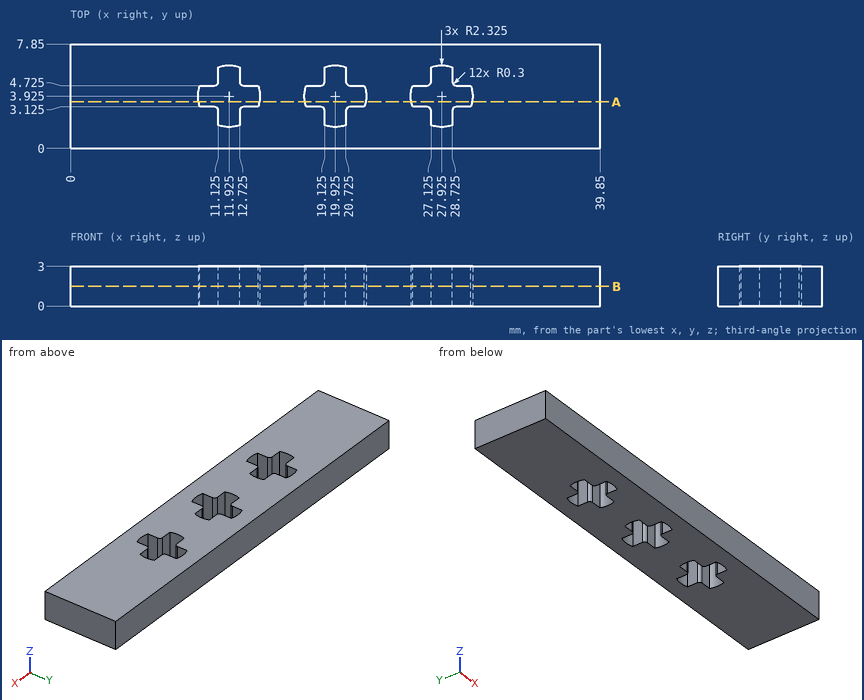
Input: dimensioned drawing with shaded views. Units: mm. Origin: part minimum x, y, z. Give positions to 0.01 mm unless a question says otherwise; leave off trailing zeros. Loops run counter-clockwise (first coordinate to the right, second up) from the corner with the lowest first, then second, coordinate; pieces in that order, holes last. Notation, with made-up numbers: M 87,68 L 138,68 A20 ccw 138,98 Z; hole C 85.25,11.5 d7. An arc over 180 degrees is marked long. Put each result on its own line as item: value.
1) Cut plane A-A, the plane y = 3.5. Return the cut outline in (x, z), plus the area to 3 significant figures.
Computed values:
outline: M 0,0 L 9.64,0 L 9.64,3 L 0,3 Z; M 14.21,0 L 17.64,0 L 17.64,3 L 14.21,3 Z; M 22.21,0 L 25.64,0 L 25.64,3 L 22.21,3 Z; M 30.21,0 L 39.85,0 L 39.85,3 L 30.21,3 Z
area: 78.4 mm^2
2) Material intervals for L1, parallel to X at y = 2.25, z = 1.4 (3 decimals); L2, parallel to X at y = 3.75, z = 0.8; L3, parallel to Y at x = 26, z = 2.35 (3 decimals), sorted ascending. Write a range as from..to.
Computed values:
L1: x = 0..11.125, 12.725..19.125, 20.725..27.125, 28.725..39.85
L2: x = 0..9.61, 14.24..17.61, 22.24..25.61, 30.24..39.85
L3: y = 0..3.125, 4.725..7.85
3) Cut plane B-B, the plane z = 1.5. Give the number of separate pieces and of enclosed holes in the cut face, plus the area to 3 significant figures.
Computed values:
separate pieces: 1
enclosed holes: 3
area: 277 mm^2
